For this review, use the dimensioned drawing (mm, ordinates from the lowest corner) and the shaded views. Coordinates: 2 decimals unless noted, no trailing zeros. Loops run counter-clockwise (first coordinate to the right, second up) from the corner with the lowest first, then second, coordinate; pieces in that order, holes last. Notation, with made-up numbers: (81, 13) - (121, 13) arc R27 ccw to (121, 37) - close; hole circle Ø9 at (33.25, 35). An arc over 180 degrees is marked (long way). Use one line per item in the form item = value. Start each with the question number.
(1) Add section B-B (x = 367). State the section outline as (y, z) points.
(2) For L1, parallel to Z at x = 54, y = 3.5, list the stretches that pass through material, from the lowest coordinate up.
(3) Clearance check with flat-ended pins moving along their axes: pin 1 Ø3 at (y, z) = (7.5, 35) entering from -X; pin 2 Ø5.5 at (x, z) = (367, 20) entering from -Y. State where each tip first meets the part, or that it passes through.
(4) Add section A-A (z = 20). State the section outline as (x, y) points, plus the area to 3 significant figures.
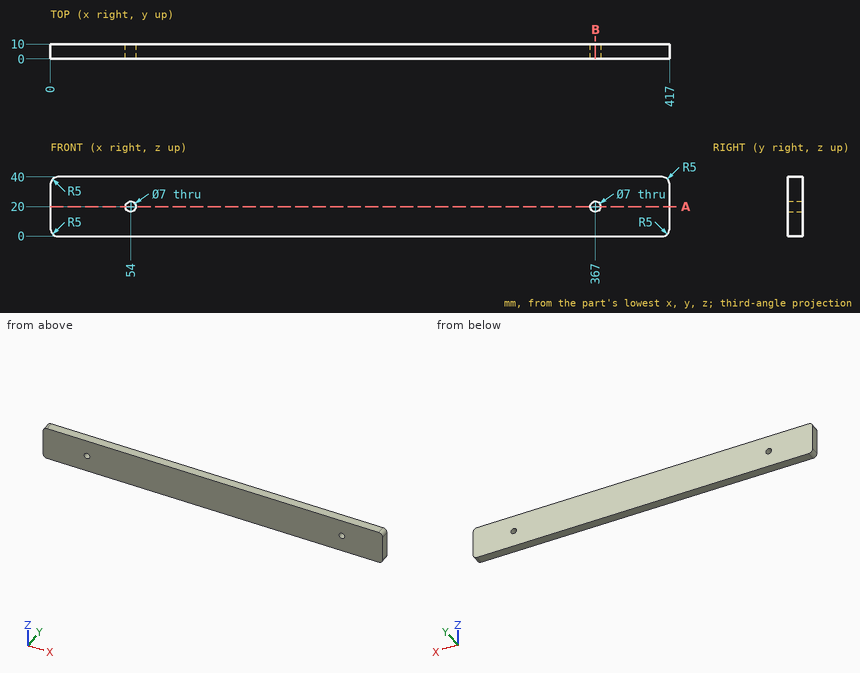
Computed values:
q1.outline = (0, 0) - (10, 0) - (10, 16.5) - (0, 16.5) - close; (0, 23.5) - (10, 23.5) - (10, 40) - (0, 40) - close
q2.L1 = 0 to 16.5, 23.5 to 40
q3.pin_1 = 0
q3.pin_2 = through
q4.outline = (0, 0) - (50.5, 0) - (50.5, 10) - (0, 10) - close; (57.5, 0) - (363.5, 0) - (363.5, 10) - (57.5, 10) - close; (370.5, 0) - (417, 0) - (417, 10) - (370.5, 10) - close
q4.area = 4,030 mm^2
